```python
from build123d import *

# Parameters (mm, degrees)
F0_W     = 2000
F0_H     = 900
F1_DEPTH = 19
F2_W     = 2000
F2_H     = 900
F2_W_2   = 1700
F2_H_2   = 600
F3_DEPTH = 19
F4_R     = 20


with BuildPart() as f1:
    # F0 (on Top) → F1 (new body)
    with BuildSketch(Plane.XY):
        with Locations((3.94921, 185.664962)):
            Rectangle(F0_W, F0_H)
    extrude(amount=F1_DEPTH)

    # F2 (on face) → F3 (join)
    with BuildSketch(Plane.XY.offset(19)):
        with Locations((3.94921, 185.664962)):
            Rectangle(F2_W, F2_H)
        with Locations((3.94921, 185.664962)):
            Rectangle(F2_W_2, F2_H_2, mode=Mode.SUBTRACT)
    extrude(amount=F3_DEPTH)

    # F4
    f4_edges = [f1.edges().sort_by_distance(p)[0] for p in [
        (1003.94921, -264.335038, 19),
        (1003.94921, 635.664962, 19),
        (-996.05079, -264.335038, 19),
        (-996.05079, 635.664962, 19),
    ]]
    fillet(f4_edges, radius=F4_R)


solid = f1.part
```
Check sheet for the modelled part. Datum: model origin and axes. Units: mm. Give positions to 0.01 mm unless a question says otherwise; leave off trailing zeros. Order: outer loops, then holes, each group sorted by start corner. A loop starts at its lowest first (then second) coordinate and runs counter-clockwise, first axis right, second up. Notation, with made-up numbers: M -4,39 L 33,39 A29 ccw 33,78 Z; hole C 56,78 d3. An arc over 180 degrees is marked long. Answer in a Markdown table with one row per item. Add a question column.
Q1. Sectioned sample at B-B, the plane z = 25. Record the boundary of the cut face in (x, y), and give its area (3 significant figures).
Q2. Release check for a two-part mould opening along Y. For faces 1 (the flat face through (-8, 190, 19)), 2 (the flat face through (-10, 635.665, 19)), 3 (the flat face through (1003.949, 180, 19)) record: released by +Y, released by -Y, zero draft, split by the parting line, or undercut.
Q3. Thickness scan on L1, parallel to Y at x = -207.5, z = 33; L2, parallel to X at y = 223, z = 29; L3, parallel to Z at x = -45.5, y = 145. Record the ranges inside material, lowest first.
Q4. Gauge pin test, flat end, axial feed: pin 1 Ø6 at (x, y) = (208, 3.5) entering from +Z. Record the tip position at first contact, or that the pin passes through.
Q5. Sectioned sample at C-C, the plane x = -423. Record the boundary of the cut face in (y, z).
Q6. Sectioned sample at A-A, the plane y = 295.5. Record the boundary of the cut face in (x, z).
Verdict:
| question | item | result |
|---|---|---|
| 1 | outline | M -996.05,-244.34 A20 ccw -976.05,-264.34 L 983.95,-264.34 A20 ccw 1003.95,-244.34 L 1003.95,615.66 A20 ccw 983.95,635.66 L -976.05,635.66 A20 ccw -996.05,615.66 Z; hole M -846.05,-114.34 L 853.95,-114.34 L 853.95,485.66 L -846.05,485.66 Z |
| 1 | area | 780,000 mm² |
| 2 | face 1 | undercut |
| 2 | face 2 | released by +Y |
| 2 | face 3 | zero draft |
| 3 | L1 | -264.34 to -114.34, 485.66 to 635.66 |
| 3 | L2 | -996.05 to -846.05, 853.95 to 1003.95 |
| 3 | L3 | 0 to 19 |
| 4 | pin 1 | z = 19 |
| 5 | outline | M -264.34,0 L 635.66,0 L 635.66,38 L 485.66,38 L 485.66,19 L -114.34,19 L -114.34,38 L -264.34,38 Z |
| 6 | outline | M -996.05,0 L 1003.95,0 L 1003.95,38 L 853.95,38 L 853.95,19 L -846.05,19 L -846.05,38 L -996.05,38 Z |
